For this review, take the finished solid that the model builds, in its own axes (mm). A direction names the side the tool comes from. Coordinates: 2 decimals unless noted, no trailing zeros. Write each loop counter-clockwise with the first axis right and the second up, starting at its lowest first coordinate (ties: lowest second). Pieces come first, ordered by that corner, then holes.
1) Insertion check: P1, Ø1.5, axis at x = 0.5, z = 2.5, coming from the +Y side; P2, Ø1.5, axis at x = 5.5, y = -1.5, coming from the +Z side; P3, Ø1.5, axis at x = -5, z = 1, coming from the -Y side. Each pin has a flat end and moves straight along its axis. Give the tip position at first contact, or say it passes through.
2) We need section C-C on z = 1.3. Write out the cut boundary in (x, y), then the cut area to 3 significant figures.
3) Mouldability with a two-part tool opening along X and no side actions: class faces 1 (the face through (0, -2, 3)), 2 (the face through (1.617, -0.67, 1.479)), 3 (the face through (-3, 0.1, 2.5)) as pulls with the +X half, pulls with the -X half, needs draft (parallel to the pull), parting line crosses it, or undercut.
4) For faces 4 (the face through (3.2, 0.1, 2)), 5 (the face through (1.5, -1.5, 0)), list the 3-axis set-ups (+Z, -Z, +X, -X, +Y, -Y) from which the entire face can be reached by the end or side of a thin tool; tool diameter is ignored.
5) We need section D-D on z = 2.4. Write out the cut boundary in (x, y), then the cut area to 3 significant figures.
6) To check wall thickness, follow line 1 along Y through (x, z) = (0, 2.2); line 2 along Y through (x, z) = (0, 1.7); line 3 along Z through (x, y) = (3.25, 1.5). State the ranges of each line that lie inside material, in increasing order.
7) We need section A-A on y = 0. Write out the cut boundary in (x, z), then the cut area to 3 significant figures.
from build123d import *

# Parameters (mm, degrees)
SKETCH1_R           = 7.5
SKETCH1_R_2         = 1.75
BOSS_EXTRUDE1_DEPTH = 2
SKETCH2_R           = 3
SKETCH2_R_2         = 1.75
BOSS_EXTRUDE2_DEPTH = 1
FILLET1_R           = 0.5


with BuildPart() as part:
    # Sketch1 → Boss-Extrude1 (new body)
    with BuildSketch(Plane.XY):
        Circle(SKETCH1_R)
        Circle(SKETCH1_R_2, mode=Mode.SUBTRACT)
    extrude(amount=BOSS_EXTRUDE1_DEPTH)

    # Sketch2 → Boss-Extrude2 (add)
    with BuildSketch(Plane.XY.offset(2)):
        Circle(SKETCH2_R)
        Circle(SKETCH2_R_2, mode=Mode.SUBTRACT)
    extrude(amount=BOSS_EXTRUDE2_DEPTH)

    # Fillet1
    fillet1_edges = [part.edges().sort_by_distance(p)[0] for p in [
        (-7.5, 0, 0),
    ]]
    fillet(fillet1_edges, radius=FILLET1_R)


solid = part.part
Result:
1. P1: stops at y = 7.5
1. P2: stops at z = 2
1. P3: stops at y = -6.18
2. outline: circle Ø15 at (0, 0); hole circle Ø3.5 at (0, 0)
2. area: 167 mm2
3. face 1: needs draft
3. face 2: undercut
3. face 3: parting line crosses it
4. face 4: +Z
4. face 5: -Z, +X, -X, +Y, -Y
5. outline: circle Ø6 at (0, 0); hole circle Ø3.5 at (0, 0)
5. area: 18.7 mm2
6. line 1: y = -3 to -1.75, 1.75 to 3
6. line 2: y = -7.5 to -1.75, 1.75 to 7.5
6. line 3: z = 0 to 2
7. outline: (-7.5, 0.5) arc R0.5 ccw to (-7, 0) - (-1.75, 0) - (-1.75, 3) - (-3, 3) - (-3, 2) - (-7.5, 2) - close; (1.75, 0) - (7, 0) arc R0.5 ccw to (7.5, 0.5) - (7.5, 2) - (3, 2) - (3, 3) - (1.75, 3) - close
7. area: 25.4 mm2
